Could you check a few things on this model? Use its own coordinates, in mm. A direction names the side the tool comes from. Coordinates: 2 decimals unless noted, no trailing zeros. Loops run counter-clockwise (first coordinate to the right, second up) from the corner with the lowest first, then second, coordinate; pieces in that order, holes last. Notation, with made-up numbers: (-37.75, 31.25) -> (-6.75, 31.25) arc R14 cw to (-6.75, 40.25) -> close; hole circle Ø7 at (10.25, 42.25). An arc over 180 degrees is marked (long way). One line per question, with ' | ' between items.
```python
from build123d import *

# Parameters (mm, degrees)
EXTRUDE_1_DEPTH     = 20
SKETCH_2_R          = 3
SKETCH_2_R_2        = 4.5
CUT_EXTRUDE_1_DEPTH = 20
SKETCH_3_R          = 3
SKETCH_3_R_2        = 4.5
CUT_EXTRUDE_2_DEPTH = 20


with BuildPart() as part:
    # 草图1 → 凸台-拉伸1 (new body)
    with BuildSketch(Plane(origin=(0, 0, 0), x_dir=(1, 0, 0), z_dir=(0, 1, 0))):
        Polygon((0, 0), (0, -90), (20, -90), (20, -20), (90, -20), (90, 0), align=None)
    extrude(amount=EXTRUDE_1_DEPTH)

    # 草图2 → 切除-拉伸1 (cut)
    with BuildSketch(Plane.ZY):
        with Locations((35, 10)):
            Circle(SKETCH_2_R)
        with Locations((50, 10)):
            Circle(SKETCH_2_R_2)
        with Locations((65, 10)):
            Circle(SKETCH_2_R)
        with Locations((80, 10)):
            Circle(SKETCH_2_R_2)
    extrude(amount=-CUT_EXTRUDE_1_DEPTH, mode=Mode.SUBTRACT)

    # 草图3 → 切除-拉伸2 (cut)
    with BuildSketch(Plane(origin=(0, 0, 0), x_dir=(-1, 0, 0), z_dir=(0, 0, -1))):
        with Locations((-35, 10)):
            Circle(SKETCH_3_R)
        with Locations((-50, 10)):
            Circle(SKETCH_3_R_2)
        with Locations((-65, 10)):
            Circle(SKETCH_3_R)
        with Locations((-80, 10)):
            Circle(SKETCH_3_R_2)
    extrude(amount=-CUT_EXTRUDE_2_DEPTH, mode=Mode.SUBTRACT)


solid = part.part
```
Q1. Please list where these lines run through material, in increasing order: L1, parallel to Z at x = 4, y = 8; L2, parallel to Y at x = 80, z = 11.5; L3, parallel to Y at x = 65, z = 10. Write a range as [from, to].
Values follow:
L1: z = [0, 32.76], [37.24, 45.97], [54.03, 62.76], [67.24, 75.97], [84.03, 90] | L2: y = [0, 5.5], [14.5, 20] | L3: y = [0, 7], [13, 20]
Q2. Imagine slicing it at D-D on y = 10. Give the number of separate pieces and of enclosed holes in the cut face, plus the area to 3 significant figures.
Values follow:
separate pieces: 9 | enclosed holes: 0 | area: 2,000 mm2
Q3. Imagine slicing it at B-B on z = 35. Write out the boundary of the cut face in (x, y).
Values follow:
outline: (0, 0) -> (20, 0) -> (20, 7) -> (0, 7) -> close; (0, 13) -> (20, 13) -> (20, 20) -> (0, 20) -> close
Q4. Imagine slicing it at C-C on x = 18. Write out the boundary of the cut face in (y, z), plus the area to 3 significant figures.
Values follow:
outline: (0, 0) -> (20, 0) -> (20, 90) -> (0, 90) -> close; hole circle Ø9 at (10, 50); hole circle Ø9 at (10, 80); hole circle Ø6 at (10, 35); hole circle Ø6 at (10, 65) | area: 1,620 mm2
Q5. Imagine slicing it at A-A on x = 65. Write out the boundary of the cut face in (y, z), plus the area to 3 significant figures.
Values follow:
outline: (0, 0) -> (7, 0) -> (7, 20) -> (0, 20) -> close; (13, 0) -> (20, 0) -> (20, 20) -> (13, 20) -> close | area: 280 mm2
Q6. For faces 1 (the face through (55, 10, 20)), 2 (the face through (10, 10, 32)), which set-ups out of +Z, -Z, +X, -X, +Y, -Y let a thin tool reach every point of the face, with its end or its side?
Values follow:
face 1: +Z, +X, +Y, -Y | face 2: +X, -X
Q7. For pin 1 (8 mm diameter, centred on y = 10, z = 65, fed in from +X), with a flat end and sliding along its axis, tell me the tip position at first contact or that it passes through.
Values follow:
pin 1: stops at x = 20
Q8. We'd pull the mould along Y, two halves only. Please class faces 3 (the face through (24, 0, 14)), 4 (the face through (24, 20, 14)), 5 (the face through (45.708, 11.352, 9.86)), 6 (the face through (10, 10, 90)): released by +Y, released by -Y, zero draft, split by the parting line, or undercut.
Values follow:
face 3: released by -Y | face 4: released by +Y | face 5: undercut | face 6: zero draft
